Geometry: final body of the model. Coordinates: model frame, mm. A direction names the side the tool comes from. Give positions to 0.01 mm unless a question says otherwise; leave off trailing zeros. Order: outer loops, then holes, each group sorted by start corner. A loop starts at its lowest first (then second) coordinate and runs counter-clockwise, first axis right, second up. Notation, with made-up numbers: (56.25, 1.5) - (69.25, 1.5) arc R34 ccw to (69.25, 38.5) - close; hole circle Ø10 at (79.25, 14.25). An arc over 180 degrees is marked (long way). Put each result on its own line as item: value. Start each with the question number.
1. Section A-A on x = 12. Return the cut outline in (y, z), plus the area to 3 significant figures.
2. First-contact query: P1, Ø3, axis at x = 16.5, z = 4, coming from the -Y side; P2, Ø0.5, axis at y = -8, z = 0.5, coming from the +X side; P3, Ø2.5, axis at x = 10, y = -5, coming from the +Z side. Flat tips, straight axial feed; report the tip coordinate or a pass-through.
3. Section C-C on y = -11.25. Return the cut outline in (x, z).
4. Ray query, line 1 along X through (y, z) = (-5.5, 2.1); line 2 along Y through (x, z) = (15.5, 2.65). Return the intervals inside material, ascending. Write a range as from..to.
5. Section B-B on y = -4. Return the cut outline in (x, z).
6. Set-up query: faces 1 (the flat face through (18.2, -5, 0.5)), 2 (the flat face through (16, -2, 0)), 3 (the flat face through (16, -1, 3)). Return all of +Z, -Z, +X, -X, +Y, -Y with unobstructed straight access to the full face (end or side cutting, diameter ignored); none if empty.
from build123d import *

# Parameters (mm, degrees)
BOSS_EXTRU_1_DEPTH      = 5
ENL_V_MAT_EXTRU_1_DEPTH = 4


with BuildPart() as part:
    # Esquisse1 → Boss.-Extru.1 (new body)
    with BuildSketch(Plane.XY):
        Polygon((0, 0), (31, 0), (31, -5), (5, -5), (5, -10), (1, -10), (1, -15), (0, -15), align=None)
    extrude(amount=BOSS_EXTRU_1_DEPTH)

    # Esquisse2 → Enlèv. mat.-Extru.1 (cut)
    with BuildSketch(Plane.XY.offset(5)):
        Polygon((1, -10), (1, -1), (31, -1), (31, -5), (5, -5), (5, -10), align=None)
    extrude(amount=-ENL_V_MAT_EXTRU_1_DEPTH, mode=Mode.SUBTRACT)


solid = part.part
Resolved:
1. outline: (-5, 0) - (0, 0) - (0, 5) - (-1, 5) - (-1, 1) - (-5, 1) - close
1. area: 9.00 mm^2
2. P1: y = -1
2. P2: x = 5
2. P3: z = 1
3. outline: (0, 0) - (1, 0) - (1, 5) - (0, 5) - close
4. line 1: 0..1
4. line 2: -1..0
5. outline: (0, 0) - (31, 0) - (31, 1) - (1, 1) - (1, 5) - (0, 5) - close
6. face 1: +Z, -Z, +X, -Y
6. face 2: -Z, +X, -X, +Y, -Y
6. face 3: +Z, +X, -Y
